Answer from the drawing. Dimensions are ordinates in mm from the lowest x, y and z of the part. Coordinates: 2 decimals unless noted, no trailing zeros. Order: outer loops, then holes, each group sorted by start corner. A loop starts at its lowest first (then second) coordinate and runs counter-clockwise, first axis right, second up. Notation, with made-up numbers: (4, 45.25) - (53, 45.25) arc R20 ccw to (53, 72.25) - close; hole circle Ø7 at (-37, 62.5). An arc over 180 degrees is marked (long way). Use a Markdown table: item, result. Add a question column.
Item 1: A flat-ended cylindrical pin translates along its axis: P1, Ø2.5, axis at y = 2.25, z = 6, coming from the +X side. Find the tip coordinate at first contact, or state that the pin passes through.
Item 2: The part is cut by section B-B, the plane y = 2.25. Give the vertices of the cut face in (x, z), then the cut area to 3 significant figures.
Item 3: Find the intervals of material crossed by line 1 along Z through (x, y) = (1.5, 2.25); line 2 along Y through (x, z) = (1.7, 6); line 3 along Z through (x, y) = (0.25, 3.2), in increasing order.
Item 4: The part is cut by section A-A, the plane z = 6. Give the vertices of the cut face in (x, y), then the cut area to 3 significant figures.
Item 5: The part is cut by section C-C, the plane x = 0.5. Give the vertices of the cut face in (y, z).
Item 6: The mould has two halves that part along Y. Classify the marked faces 1, 2, 3 and 4: released by +Y, released by -Y, zero draft, split by the parting line, or undercut.
Item 7: The part is cut by section D-D, the plane z = 21.75. Give the vertices of the cut face in (x, y).
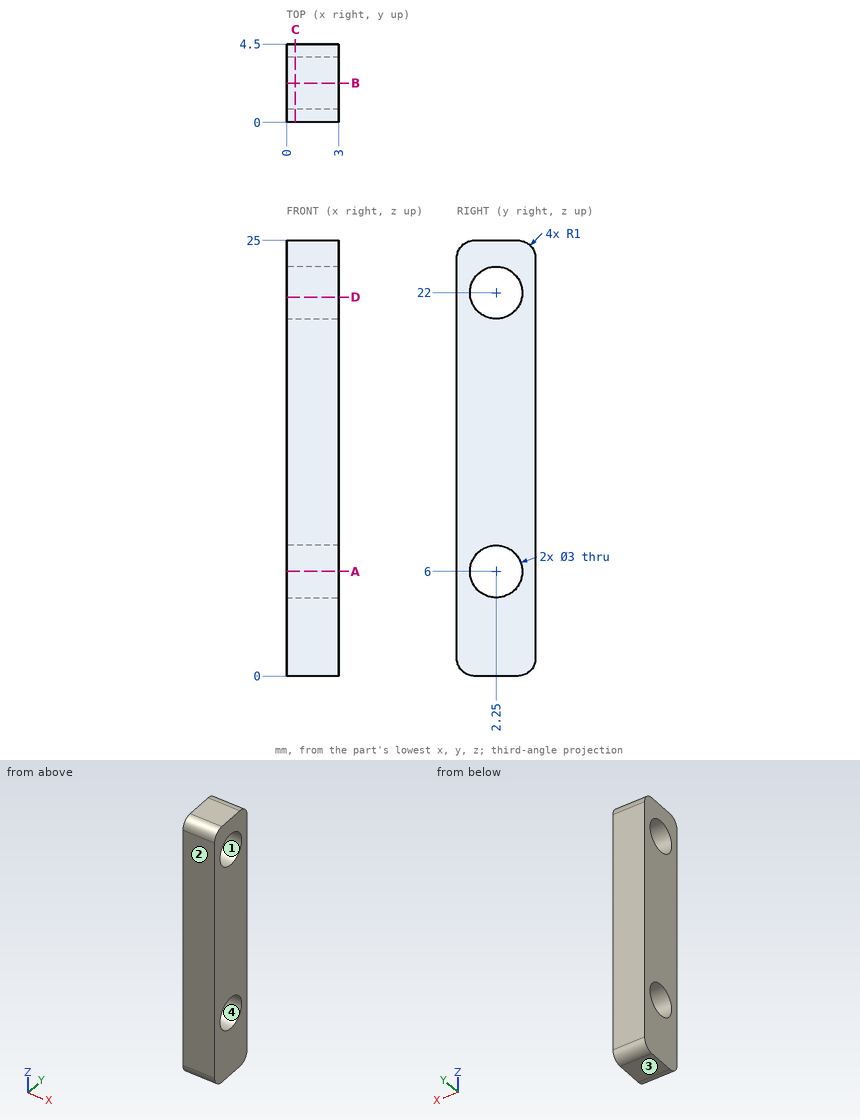
Solution:
| question | item | result |
|---|---|---|
| 1 | P1 | passes through |
| 2 | outline | (0, 0) - (3, 0) - (3, 4.5) - (0, 4.5) - close; (0, 7.5) - (3, 7.5) - (3, 20.5) - (0, 20.5) - close; (0, 23.5) - (3, 23.5) - (3, 25) - (0, 25) - close |
| 2 | area | 57.0 mm2 |
| 3 | line 1 | z = 0 to 4.5, 7.5 to 20.5, 23.5 to 25 |
| 3 | line 2 | y = 0 to 0.75, 3.75 to 4.5 |
| 3 | line 3 | z = 0 to 4.84, 7.16 to 20.84, 23.16 to 25 |
| 4 | outline | (0, 0) - (3, 0) - (3, 0.75) - (0, 0.75) - close; (0, 3.75) - (3, 3.75) - (3, 4.5) - (0, 4.5) - close |
| 4 | area | 4.50 mm2 |
| 5 | outline | (0, 1) arc R1 ccw to (1, 0) - (3.5, 0) arc R1 ccw to (4.5, 1) - (4.5, 24) arc R1 ccw to (3.5, 25) - (1, 25) arc R1 ccw to (0, 24) - close; hole circle Ø3 at (2.25, 6); hole circle Ø3 at (2.25, 22) |
| 6 | face 1 | undercut |
| 6 | face 2 | released by -Y |
| 6 | face 3 | zero draft |
| 6 | face 4 | undercut |
| 7 | outline | (0, 0) - (3, 0) - (3, 0.77) - (0, 0.77) - close; (0, 3.73) - (3, 3.73) - (3, 4.5) - (0, 4.5) - close |
